Source: CAD feature listing. Evaluate the final solid. Frame: model axes, mm. A direction names the side the tool comes from. Give positions to 0.01 mm unless a question says otherwise; leave off trailing zeros. Order: outer loops, then holes, each group sorted by start corner. A loop starts at its lowest first (then second) coordinate and runs counter-clockwise, first axis right, second up. Notation, with made-up numbers: M 87,-14.5 L 116,-14.5 A15 cw 116,11.5 Z; hole C 73.5,0.25 d4. An arc over 180 degrees is marked long. Answer as a JSON object with one key per item and string values. Group by question number.
1. Section query C-C (y = 12). Output: boundary loops of the cut face in (x, z), plus the area to 3 significant figures.
2. Pin query (flat end, axial travel): P1, Ø6, axis at y = -14, z = 8, coming from the +X side; P2, Ø13, axis at y = -9.5, z = 41, coming from the -X side; P3, Ø3.5, axis at y = -16.5, z = 3, coming from the -X side. Return the tip coordinate at first contact, or that it passes through.
3. Pull-direction query (Z, two-part tool) for faces 1 (the flat face through (7, -22, 25)), 2 (the cylindrical face through (9, -5.9, 51.3)); classes: +Z half, -Z half, draft (parallel to the pull), parting line (faces both ways), or undercut.
4. Set-up query: faces 3 (the flat face through (31, -6.5, 53)), 4 (the cylindrical face through (48.407, 12.334, 27.115)), 5 (the flat face through (21, -10, 5)), 6 (the flat face through (40, -13, 27)). Return all of +Z, -Z, +X, -X, +Y, -Y with unobstructed straight access to the full face (end or side cutting, diameter ignored); none if empty.
5. Material intervals for L1, parallel to X at y = 12, z = 17; L2, parallel to Z at x = 17, y = -19.5; L3, parallel to Y at x = 16.5, z = 24, sorted ascending. Write a range as [from, to].
6. Section query A-A (x = 12). Output: boundary loops of the cut face in (y, z).
7. Section query B-B (z = 2.5). Output: boundary loops of the cut face in (x, y), plus the area to 3 significant figures.
8. Section query D-D (x = 56). Output: boundary loops of the cut face in (y, z), plus the area to 3 significant figures.
from build123d import *

# Parameters (mm, degrees)
ESQUISSE1_W             = 70
ESQUISSE1_H             = 24
BOSS_EXTRU_1_DEPTH      = 55
ESQUISSE2_R             = 7.6
ENL_V_MAT_EXTRU_1_DEPTH = 93.200867675
BOSS_EXTRU_3_DEPTH      = 21
ESQUISSE9_W             = 33
ESQUISSE9_H             = 55
BOSS_EXTRU_4_DEPTH      = 5
ESQUISSE10_R            = 1.5
ENL_V_MAT_EXTRU_4_DEPTH = 4
ESQUISSE11_W            = 5.5
ESQUISSE11_H            = 8
ENL_V_MAT_EXTRU_5_DEPTH = 10


with BuildPart() as part:
    # Esquisse1 → Boss.-Extru.1 (new body)
    with BuildSketch(Plane.XY):
        with Locations((35, 12)):
            Rectangle(ESQUISSE1_W, ESQUISSE1_H)
    extrude(amount=BOSS_EXTRU_1_DEPTH)

    # Esquisse2 → Enlèv. mat.-Extru.1 (cut, through all)
    with BuildSketch(Plane.XY):
        with Locations((56, 12)):
            Circle(ESQUISSE2_R)
        with Locations((12, 12)):
            Circle(ESQUISSE2_R)
    extrude(amount=ENL_V_MAT_EXTRU_1_DEPTH, mode=Mode.SUBTRACT)

    # Esquisse6 → Boss.-Extru.3 (add)
    with BuildSketch(Plane.XZ):
        Polygon((7, 0), (40, 0), (40, 55), (7, 55), (7, 50), (35, 50), (35, 5), (7, 5), align=None)
    extrude(amount=BOSS_EXTRU_3_DEPTH)

    # Esquisse9 → Boss.-Extru.4 (add)
    with BuildSketch(Plane.XZ.offset(21)):
        with Locations((23.5, 27.5)):
            Rectangle(ESQUISSE9_W, ESQUISSE9_H)
    extrude(amount=BOSS_EXTRU_4_DEPTH)

    # Esquisse10 → Enlèv. mat.-Extru.4 (cut)
    with BuildSketch(Plane.ZY.offset(-7)):
        with Locations((52.5, -16)):
            Circle(ESQUISSE10_R)
        with Locations((52.5, -5)):
            Circle(ESQUISSE10_R)
        with Locations((2.5, -16)):
            Circle(ESQUISSE10_R)
        with Locations((2.5, -5)):
            Circle(ESQUISSE10_R)
    extrude(amount=-ENL_V_MAT_EXTRU_4_DEPTH, mode=Mode.SUBTRACT)

    # Esquisse11 → Enlèv. mat.-Extru.5 (cut)
    with BuildSketch(Plane.XY.offset(55)):
        with Locations((31.25, -10.5)):
            Rectangle(ESQUISSE11_W, ESQUISSE11_H)
    extrude(amount=-ENL_V_MAT_EXTRU_5_DEPTH, mode=Mode.SUBTRACT)


solid = part.part
Answer sheet:
{
 "1": {"outline": "M 0,0 L 4.4,0 L 4.4,55 L 0,55 Z; M 19.6,0 L 48.4,0 L 48.4,55 L 19.6,55 Z; M 63.6,0 L 70,0 L 70,55 L 63.6,55 Z", "area": "2,180 mm^2"},
 "2": {"P1": "x = 40", "P2": "x = 35", "P3": "x = 7"},
 "3": {"face 1": "draft", "face 2": "undercut"},
 "4": {"face 3": "+Z", "face 4": "+Z, -Z", "face 5": "-X", "face 6": "+Z, -Z, +X, -Y"},
 "5": {"L1": "[0, 4.4], [19.6, 48.4], [63.6, 70]", "L2": "[0, 5], [50, 55]", "L3": "[-26, -21], [0, 5.88], [18.12, 24]"},
 "6": {"outline": "M -26,0 L 4.4,0 L 4.4,55 L -26,55 Z; M 19.6,0 L 24,0 L 24,55 L 19.6,55 Z; hole M -21,5 L 0,5 L 0,50 L -21,50 Z"},
 "7": {"outline": "M 0,0 L 7,0 L 7,-3.5 L 11,-3.5 L 11,-6.5 L 7,-6.5 L 7,-14.5 L 11,-14.5 L 11,-17.5 L 7,-17.5 L 7,-26 L 40,-26 L 40,0 L 70,0 L 70,24 L 0,24 Z; hole C 12,12 d15.2; hole C 56,12 d15.2", "area": "2,150 mm^2"},
 "8": {"outline": "M 0,0 L 4.4,0 L 4.4,55 L 0,55 Z; M 19.6,0 L 24,0 L 24,55 L 19.6,55 Z", "area": "484 mm^2"}
}
